Design review of the part built by this model. Coordinates are the model's own, in mm. Give positions to 0.01 mm unless a question says otherwise; leave off trailing zeros. Write each loop counter-clockwise with the first axis right and the second up, starting at its lowest first coordinate (ties: lowest second). Pieces come first, ordered by that corner, then holes. Notation, with made-up numbers: M -29,11.5 L 30,11.5 A17 ccw 30,22.5 Z; hole C 55,62.25 d8. An arc over 180 degrees is marked long. Answer in a Markdown table with one row per item.
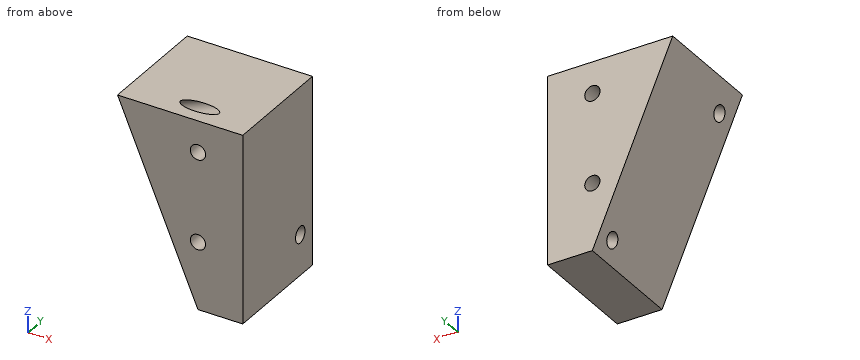
Autodesk Inventor part; units mm, degrees
ref_plane "YZ Plane" through (0, 0, 0) normal (1, 0, 0) x (0, 1, 0)
ref_plane "XZ Plane" through (0, 0, 0) normal (0, 1, 0) x (-1, 0, 0)
ref_plane "XY Plane" through (0, 0, 0) normal (0, 0, 1) x (1, 0, 0)
sketch "Sketch1" plane through (0, 0, 0) normal (0, 1, 0) x (-1, 0, 0)
  line L0 (0, 0) -> (17.7417, 0)
  line L1 (17.7417, 0) -> (6.35, -26.6689)
  line L2 (6.35, -26.6689) -> (0, -26.6689)
  line L3 (0, -26.6689) -> (0, 0)
  dimension "d0" = 23.13
  dimension "d1" = 29
  dimension "d2" = 6.35
extrude "Extrusion1" add sketch "Sketch1" along normal blind 16
sketch "Sketch2" plane through (-17.7417, 0, 0) normal (-0.9196159, 0, -0.3928187) x (-0.3928187, 0, 0.9196159)
  line L0 (-29, 16) -> (0, 16) construction
  line L1 (-29, 0) -> (-29, 16) construction
  line L2 (0, 0) -> (-29, 0) construction
  line L3 (0, 0) -> (0, 16) construction
  point P0 (-6.9693, 0)
  point P1 (-3.8988, 2.8114)
  point P2 (-26.2, 13.2)
  dimension "d5" = 2.8
  dimension "d6" = 2.8
  dimension "d26" = 22.3012
  dimension "d27" = 10.3886
hole "Hole1" at (-16.2102, 2.8114, -3.5854) at (-7.4499, 13.2, -24.0939) direction (0.9196159, 0, 0.3928187) diameter 2.159 end through all
sketch "Sketch3" plane through (0, 16, 0) normal (0, 1, 0) x (1, 0, 0)
  line L0 (-17.7417, 0) -> (0, 0) construction
  line L1 (-6.35, 0) -> (-6.35, 26.6689) construction
  line L2 (0, 26.6689) -> (-6.35, 26.6689) construction
  line L3 (0, 0) -> (0, 26.6689) construction
  point P0 (-6.35, 4.445)
  point P1 (-6.35, 17.1439)
  dimension "d16" = 6.35
  dimension "d17" = 4.445
  dimension "d18" = 9.525
  dimension "d28" = 12.6989
hole "Hole2" at (-6.35, 16, -4.445) at (-6.35, 16, -17.1439) direction (0, -1, 0) diameter 2.159 end through all
properties part number "Microswitch_Bracket" material "ABS Plastic"
1) Add section A-A (y = 8.5). Count the separate pieces of the cut face and the enclosed holes in it, and give its area (3 significant figures).
Geometry says:
| item | result |
|---|---|
| separate pieces | 1 |
| enclosed holes | 2 |
| area | 314 mm^2 |
2) Add section B-B (z = -9.25). Write out the cut boundary in (x, y).
Geometry says:
| item | result |
|---|---|
| outline | M -13.79,0 L 0,0 L 0,16 L -13.79,16 Z |
3) Insertion check: P1, Ø8, axis at y = 14, z = -13.5, coming from the -X side; P2, Ø1.5, axis at y = 4.5, z = -20, coming from the -X side. Each pin has a flat end and moves straight along its axis. Give the tip position at first contact, or say it passes through.
Geometry says:
| item | result |
|---|---|
| P1 | x = -13.68 |
| P2 | x = -9.52 |
4) To check wall thickness, follow probe 1 along Z at (x, y) = (-7, 10.25); probe 2 along X at (y, z) = (6.75, -18); probe 3 along X at (y, z) = (6.5, -17.5). State the ranges of each line that lie inside material, in increasing order. Write a range as [from, to].
Geometry says:
| item | result |
|---|---|
| probe 1 | [-25.15, -18.01], [-16.28, -5.31], [-3.58, 0] |
| probe 2 | [-10.05, -7.01], [-5.69, 0] |
| probe 3 | [-10.27, -7.37], [-5.33, 0] |
